Could you check a few things on this drawing? It's one solid part, dimensions in mm from its lowest x, y, z. Coordinates: 2 decimals unless noted, no trailing zeros. Write each loop counter-clockwise with the first axis right and the second up, starting at its lowest first coordinate (ties: lowest second). Pieces come first, ordered by that corner, then holes.
Item 1: If we mould it in two halves opening along Z, with no side actions, what happens to the marked faces 1, 2 and 3? For each: pulls with the +Z half, pulls with the -Z half, needs draft (parallel to the pull), parting line crosses it, or undercut.
Item 2: I'm going to push flat-ended pins straight in: P1, Ø5, axis at x = 16, z = 5, coming from the +Y side; P2, Ø1.5, axis at y = 11, z = 14.5, coming from the -X side; P3, Ø4, axis at y = 8, z = 15, coming from the -X side; P4, Ø8, axis at y = 8.5, z = 11.5, coming from the -X side. Where does each tip first touch, or does it pass through?
Item 3: I want a section at B-B (y = 9.75). Please give me the cut outline in (x, z).
Item 4: I want a section at C-C (y = 17). Please give me the cut outline in (x, z).
Item 5: I want a section at A-A (x = 10). Please give me the cut outline in (y, z).
Item 6: Please list where these lines run through material, in increasing order: line 1 (Z direction, x = 13.25, y = 2.75) (1 decimal); line 2 (X direction, y = 16.5, z = 12.25) (1 decimal); line 3 (Z direction, x = 6.25, y = 3.75) (1 decimal).
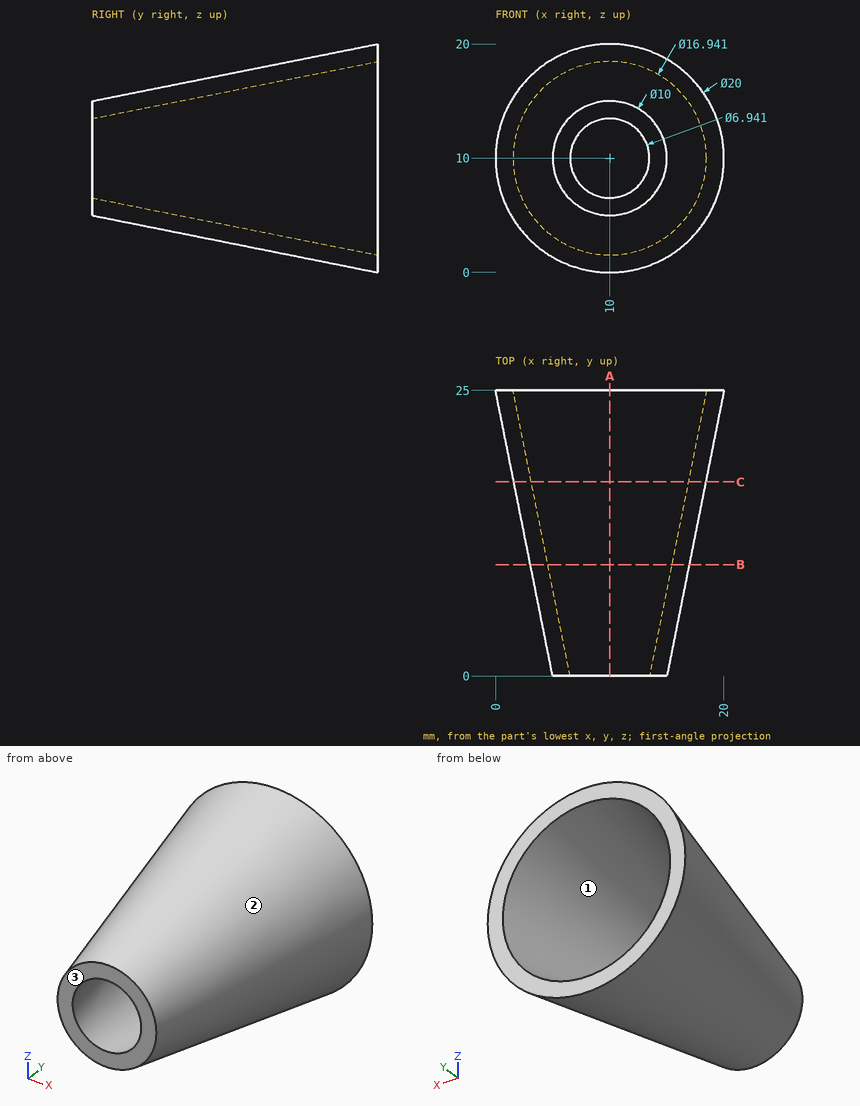
Answer:
1. face 1: undercut
1. face 2: parting line crosses it
1. face 3: needs draft
2. P1: stops at y = 25
2. P2: stops at x = 3.82
2. P3: stops at x = 4.03
2. P4: stops at x = 2.54
3. outline: circle Ø13.9 at (10, 10); hole circle Ø10.84 at (10, 10)
4. outline: circle Ø16.8 at (10, 10); hole circle Ø13.74 at (10, 10)
5. outline: (0, 5) - (25, 0) - (25, 1.53) - (0, 6.53) - close; (0, 13.47) - (25, 18.47) - (25, 20) - (0, 15) - close
6. line 1: z = 5.5 to 7.6, 12.4 to 14.5
6. line 2: x = 2 to 3.6, 16.4 to 18
6. line 3: z = 5.6 to 8.1, 11.9 to 14.4
